Source: CAD feature listing. Evaluate the final solid. Frame: model axes, mm. A direction names the side the tool comes from. Round coordinates to 2 decimals unless told otherwise and drop trailing zeros. Loops run counter-clockwise (first coordinate to the right, second up) from the corner with the lowest first, then second, coordinate; pieces in that order, holes last. Notation, with made-up numbers: M 56.25,10.25 L 71.25,10.25 A22 cw 71.25,38.25 Z; hole C 72.5,38 d11. An arc over 180 degrees is marked long. Write each question's results on one line, items separated by ' | '. Start each with the question number.
1. Section D-D on x = 0. Output: boundary loops of the cut face in (y, z).
2. Section B-B on z = -6. Output: boundary loops of the cut face in (x, y), and give its area (3 significant figures).
3. Draft query along X for faces 4 (the flat face through (-1, 40, 29)), 5 (the cylindrical face through (-32.64, 32.16, 6.89)), 6 (the flat face through (42.5, 20, -10)). Return one class per face: released by +X, released by -X, zero draft, split by the parting line, or undercut.
4. Ray query, line 1 (Y direction, x = -35, z = 22.5); line 2 (Z direction, x = 0, y = 24.5); line 3 (X direction, y = 12, z = 11). Return the intervals inside material, ascending.
5. Section C-C on x = 35. Output: boundary loops of the cut face in (y, z), and give its area (3 significant figures).
6. Contact query for flat-ended pins moving along their axis: pin 1 Ø6 at (x, y) = (13, 28) entering from +Z; pin 2 Ø8.5 at (x, y) = (-35, 30) entering from -Z; pin 3 Ø8.5 at (x, y) = (-15.5, 20.5) entering from +Z; pin 4 Ø5 at (x, y) = (35, 30) entering from -Z. Output: stop coordinate, or through.
7. Set-up query: faces 1 (the flat face through (42.5, 20, 7)), 2 (the flat face through (-9.91, 19.72, 32.14)), 3 (the flat face through (-42.5, 20, -3)). Return all of +Z, -Z, +X, -X, +Y, -Y with unobstructed straight access to the full face (end or side cutting, diameter ignored); none if empty.
8. Section A-A on x = -35. Output: boundary loops of the cut face in (y, z), and give its area (3 significant figures).
from build123d import *

# Parameters (mm, degrees)
CROQUIS1_R              = 26
SALIENTE_EXTRUIR1_DEPTH = 40
CROQUIS2_R              = 3.2
CORTAR_EXTRUIR1_DEPTH   = 67.5
CORTAR_EXTRUIR2_REACH   = 89.5
CROQUIS3_W              = 1.6
CROQUIS3_H              = 40


with BuildPart() as part:
    # Croquis1 → Saliente-Extruir1 (new body)
    with BuildSketch(Plane(origin=(0, 0, 0), x_dir=(1, 0, 0), z_dir=(0, 1, 0))):
        Polygon((-42.5, 18.75), (-42.5, -13.75), (-45, -16.25), (-45, -31.25), (-43, -33.25), (-23, -33.25), (-23, -33.05), (-21.2, -31.25), (-10.8, -31.25), (-9, -33.05), (-9, -33.25), (9, -33.25), (9, -33.05), (10.8, -31.25), (21.2, -31.25), (23, -33.05), (23, -33.25), (43, -33.25), (45, -31.25), (45, -16.25), (42.5, -13.75), (42.5, 18.75), (27.1, 18.75), (14, 33.25), (-14, 33.25), (-27.1, 18.75), align=None)
        Circle(CROQUIS1_R, mode=Mode.SUBTRACT)
    extrude(amount=SALIENTE_EXTRUIR1_DEPTH)

    # Croquis2 → Cortar-Extruir1 (cut, through all)
    with BuildSketch(Plane(origin=(0, 0, -33.25), x_dir=(-1, 0, 0), z_dir=(0, 0, -1))):
        with Locations((-35, 30)):
            Circle(CROQUIS2_R)
        with Locations((-35, 10)):
            Circle(CROQUIS2_R)
        with Locations((35, 10)):
            Circle(CROQUIS2_R)
        with Locations((35, 30)):
            Circle(CROQUIS2_R)
    extrude(amount=-CORTAR_EXTRUIR1_DEPTH, mode=Mode.SUBTRACT)

    # Croquis3 → Cortar-Extruir2 (cut, up to next)
    with BuildSketch(Plane(origin=(42.5, 0, 0), x_dir=(0, 0, -1), z_dir=(1, 0, 0)), mode=Mode.PRIVATE) as cortar_extruir2_sk1:
        with Locations((-0.05, 20)):
            Rectangle(CROQUIS3_W, CROQUIS3_H)
    cortar_extruir2_tool1 = extrude(cortar_extruir2_sk1.sketch, amount=-CORTAR_EXTRUIR2_REACH, mode=Mode.PRIVATE) & part.part
    add(cortar_extruir2_tool1.solids().sort_by_distance((42.5, 20, 0.05))[0], mode=Mode.SUBTRACT)


solid = part.part
Taken from the geometry:
1) outline: M 0,-33.25 L 40,-33.25 L 40,-26 L 0,-26 Z; M 0,26 L 40,26 L 40,33.25 L 0,33.25 Z
2) outline: M -42.5,0 L -25.3,0 L -25.3,40 L -42.5,40 Z; M 25.3,0 L 42.5,0 L 42.5,40 L 25.3,40 Z; hole C -35,10 d6.4; hole C -35,30 d6.4; hole C 35,10 d6.4; hole C 35,30 d6.4 | area: 1,250 mm^2
3) face 4: zero draft | face 5: undercut | face 6: released by +X
4) line 1: 0 to 6.8, 13.2 to 26.8, 33.2 to 40 | line 2: -33.25 to -26, 26 to 33.25 | line 3: -42.5 to -37.5, -32.5 to -23.56, 23.56 to 32.5, 37.5 to 42.5
5) outline: M 0,-18.75 L 6.8,-18.75 L 6.8,-0.75 L 0,-0.75 Z; M 0,0.85 L 6.8,0.85 L 6.8,33.25 L 0,33.25 Z; M 13.2,-18.75 L 26.8,-18.75 L 26.8,-0.75 L 13.2,-0.75 Z; M 13.2,0.85 L 26.8,0.85 L 26.8,33.25 L 13.2,33.25 Z; M 33.2,-18.75 L 40,-18.75 L 40,-0.75 L 33.2,-0.75 Z; M 33.2,0.85 L 40,0.85 L 40,33.25 L 33.2,33.25 Z | area: 1,370 mm^2
6) pin 1: z = 32.05 | pin 2: z = -18.75 | pin 3: z = 31.25 | pin 4: through
7) face 1: -Z, +X, +Y, -Y | face 2: +Z, +Y, -Y | face 3: -Z, -X, +Y, -Y
8) outline: M 0,-18.75 L 6.8,-18.75 L 6.8,33.25 L 0,33.25 Z; M 13.2,-18.75 L 26.8,-18.75 L 26.8,33.25 L 13.2,33.25 Z; M 33.2,-18.75 L 40,-18.75 L 40,33.25 L 33.2,33.25 Z | area: 1,410 mm^2
